Source: CAD feature listing. Evaluate the final solid. Frame: model axes, mm. A direction names the side the tool comes from. Give positions to 0.01 mm unless a question says otherwise; leave off trailing zeros. Loops run counter-clockwise (first coordinate to the right, second up) from the corner with the lowest first, then second, coordinate; pieces in that order, holes last. Notation, with made-up numbers: (15.25, 28.25) - (58.25, 28.25) arc R15 ccw to (58.25, 54.25) - close; hole circle Ø3 at (77.25, 88.25). An arc over 180 degrees is marked (long way). Put each result on its own line as item: value.
```python
from build123d import *

# Parameters (mm, degrees)
BOSS_EXTRUDE1_DEPTH = 5
SKETCH2_R           = 1.6
CUT_EXTRUDE1_DEPTH  = 3
BOSS_EXTRUDE2_DEPTH = 12
SKETCH8_R           = 1.5
CUT_EXTRUDE2_DEPTH  = 3
FILLET1_R           = 1
SKETCH9_W           = 6
SKETCH9_H           = 3
BOSS_EXTRUDE3_DEPTH = 5
SKETCH12_W          = 3
SKETCH12_H          = 5
CUT_EXTRUDE4_DEPTH  = 17
SKETCH14_W          = 4
SKETCH14_H          = 4
BOSS_EXTRUDE5_DEPTH = 6
FILLET3_R           = 4
FILLET4_R           = 4
BOSS_EXTRUDE6_DEPTH = 5


with BuildPart() as part:
    # Sketch1 → Boss-Extrude1 (new body)
    with BuildSketch(Plane(origin=(0, 0, 0), x_dir=(1, 0, 0), z_dir=(0, 1, 0))):
        Polygon((0, 0), (20, 0), (45, 12), (45, 22), (-25, 22), (-25, 12), align=None)
    extrude(amount=BOSS_EXTRUDE1_DEPTH)

    # Sketch2 → Cut-Extrude1 (cut)
    with BuildSketch(Plane(origin=(0, 5, 0), x_dir=(1, 0, 0), z_dir=(0, 1, 0))):
        with Locations(Location((4, 6, 0), (0, 0, 270))):
            Circle(SKETCH2_R)
        with Locations(Location((16, 6, 0), (0, 0, 90))):
            Circle(SKETCH2_R)
    extrude(amount=-CUT_EXTRUDE1_DEPTH, mode=Mode.SUBTRACT)

    # Sketch3 → Boss-Extrude2 (add)
    with BuildSketch(Plane(origin=(0, 5, 0), x_dir=(1, 0, 0), z_dir=(0, 1, 0))):
        with BuildLine():
            Line((-1.313075459, 8.787692444), (-14.45873126, 6.940191005))
            Line((-14.45873126, 6.940191005), (-25, 12))
            Line((-25, 12), (-25, 22))
            Line((-25, 22), (-22, 22))
            Line((-22, 22), (-22, 13.88770191))
            Line((-22, 13.88770191), (-13.978151779, 10.037214764))
            Line((-13.978151779, 10.037214764), (-3.068994172, 11.57039688))
            ThreePointArc((-3.068994172, 11.57039688), (0.071487045, 14.097332027), (4, 15))
            Line((4, 15), (16, 15))
            ThreePointArc((16, 15), (19.928512955, 14.097332027), (23.068994172, 11.57039688))
            Line((23.068994172, 11.57039688), (33.978151779, 10.037214764))
            Line((33.978151779, 10.037214764), (42, 13.88770191))
            Line((42, 13.88770191), (42, 22))
            Line((42, 22), (45, 22))
            Line((45, 22), (45, 12))
            Line((45, 12), (34.45873126, 6.940191005))
            Line((34.45873126, 6.940191005), (21.313075459, 8.787692444))
            ThreePointArc((21.313075459, 8.787692444), (19.104339329, 11.134498742), (16, 12))
            Line((16, 12), (4, 12))
            ThreePointArc((4, 12), (0.895660671, 11.134498742), (-1.313075459, 8.787692444))
        make_face()
    extrude(amount=BOSS_EXTRUDE2_DEPTH)

    # Sketch6 → Revolve1 (revolve)
    with BuildSketch(Plane.XY.offset(-6), mode=Mode.PRIVATE) as revolve1_sk:
        Polygon((2.4, 5), (2.4, 7), (1.4, 5), align=None)
    revolve(revolve1_sk.sketch.rotate(Axis((4, 5, -6), (0, 1, 0)), 270), axis=Axis((4, 5, -6), (0, 1, 0)))

    # Sketch7 → Revolve2 (revolve)
    with BuildSketch(Plane.XY.offset(-6), mode=Mode.PRIVATE) as revolve2_sk:
        Polygon((14.4, 5), (14.4, 7), (13.4, 5), align=None)
    revolve(revolve2_sk.sketch.rotate(Axis((16, 5, -6), (0, 1, 0)), 270), axis=Axis((16, 5, -6), (0, 1, 0)))

    # Sketch8 → Cut-Extrude2 (cut)
    with BuildSketch(Plane.XY.offset(-12)):
        with Locations((10, 11)):
            Circle(SKETCH8_R)
    extrude(amount=-CUT_EXTRUDE2_DEPTH, mode=Mode.SUBTRACT)

    # Fillet1
    fillet1_edges = [part.edges().sort_by_distance(p)[0] for p in [
        (8.5, 11, -15),
        (8.5, 11, -12),
    ]]
    fillet(fillet1_edges, radius=FILLET1_R)

    # Sketch9 → Boss-Extrude3 (add)
    with BuildSketch(Plane(origin=(0, 17, 0), x_dir=(1, 0, 0), z_dir=(0, 1, 0))):
        with Locations((10, 13.5)):
            Rectangle(SKETCH9_W, SKETCH9_H)
    extrude(amount=BOSS_EXTRUDE3_DEPTH)

    # Sketch12 → Cut-Extrude4 (cut)
    with BuildSketch(Plane(origin=(0, 17, 0), x_dir=(1, 0, 0), z_dir=(0, 1, 0))):
        with Locations((-23.5, 16.5)):
            Rectangle(SKETCH12_W, SKETCH12_H)
        with Locations((43.5, 16.5)):
            Rectangle(SKETCH12_W, SKETCH12_H)
    extrude(amount=-CUT_EXTRUDE4_DEPTH, mode=Mode.SUBTRACT)

    # Sketch14 → Boss-Extrude5 (add)
    with BuildSketch(Plane(origin=(0, 5, 0), x_dir=(1, 0, 0), z_dir=(0, 1, 0))):
        with Locations((34, 20)):
            Rectangle(SKETCH14_W, SKETCH14_H)
        with Locations((-14, 20)):
            Rectangle(SKETCH14_W, SKETCH14_H)
    extrude(amount=BOSS_EXTRUDE5_DEPTH)

    # Fillet3
    fillet3_edges = [part.edges().sort_by_distance(p)[0] for p in [
        (32, 8, -18),
    ]]
    fillet(fillet3_edges, radius=FILLET3_R - 0.0001)  # a hair under: the kernel refuses the full size

    # Fillet4
    fillet4_edges = [part.edges().sort_by_distance(p)[0] for p in [
        (-12, 8, -18),
    ]]
    fillet(fillet4_edges, radius=FILLET4_R - 0.0001)  # a hair under: the kernel refuses the full size

    # Sketch15 → Boss-Extrude6 (add)
    with BuildSketch(Plane(origin=(0, 5, 0), x_dir=(1, 0, 0), z_dir=(0, 1, 0))):
        Polygon((-16, 22), (-21, 29), (-1, 29), (-6, 22), align=None)
        Polygon((36, 22), (26, 22), (21, 29), (41, 29), align=None)
    extrude(amount=-BOSS_EXTRUDE6_DEPTH)


solid = part.part
```
1) Pin query (flat end, axial travel): P1, Ø3.5, axis at x = -24, z = -21, coming from the +Y side; P2, Ø1, axis at x = 20, y = 16.5, coming from the +Z side; P3, Ø3.5, axis at x = 20, z = -6.5, coming from the +Y side. Return the tip coordinate at first contact, or that it passes through.
Check result:
P1: y = 17
P2: z = -9.97
P3: y = 5.64
2) Section query C-C, the plane x = -18. Output: boundary loops of the cut face in (y, z), plus the area to 3 significant figures.
Check result:
outline: (0, -29) - (5, -29) - (5, -24.8) - (0, -24.8) - close; (0, -22) - (5, -22) - (5, -11.97) - (17, -11.97) - (17, -8.64) - (0, -8.64) - close
area: 128 mm²
3) Material intervals for line 1 along X through (y, z) = (5.4, -6); line 2 along Z through (x, y) = (4, 4.25); line 3 along X through (y, z) = (14.75, -13), sorted ascending. Write a range as [from, to].
Check result:
line 1: [1.6, 2.4], [5.6, 6.4], [13.6, 14.4], [17.6, 18.4]
line 2: [-22, -7.6], [-4.4, 0]
line 3: [-25, -20.15], [-1.66, 21.66], [40.15, 45]
4) Access query for faces 1 (the flat face through (37.933, 10.916, -11.936)), 2 (the flat face through (-24, 9, -19)), 3 (the flat face through (-14, 11, -20)), 4 (the flat face through (29, 17, -10)), 5 (the flat face through (31, 3, -29)). Directions: +Z, -Z, +X, -X, +Y, -Y. A direction counts if a zero-diameter tool reaches every point of the face in a straight line with its end or side. Return the directions, or none.
Check result:
face 1: +Y
face 2: -X, +Y, -Y
face 3: -Z, +Y
face 4: +Z, -Z, +X, +Y
face 5: -Z, +X, -X, +Y, -Y
5) Section query D-D, the plane z = -6. Output: boundary loops of the cut face in (x, y), plus the area to 3 significant figures.
Check result:
outline: (-12.5, 0) - (32.5, 0) - (32.5, 5) - (18.6, 5) - (17.6, 7) - (17.6, 2) - (14.4, 2) - (14.4, 7) - (13.4, 5) - (6.6, 5) - (5.6, 7) - (5.6, 2) - (2.4, 2) - (2.4, 7) - (1.4, 5) - (-12.5, 5) - close
area: 210 mm²
6) Section query B-B, the plane z = -23. Output: boundary loops of the cut face in (x, y).
Check result:
outline: (-16.71, 0) - (-5.29, 0) - (-5.29, 5) - (-16.71, 5) - close; (25.29, 0) - (36.71, 0) - (36.71, 5) - (25.29, 5) - close
7) Section query A-A, the plane y = 15.75. Output: boundary loops of the cut face in (x, z), plus the area to 3 significant figures.
Check result:
outline: (-25, -22) - (-22, -22) - (-22, -19) - (-25, -19) - close; (-25, -14) - (-22, -14) - (-22, -13.89) - (-13.98, -10.04) - (-3.07, -11.57) arc R9 ccw to (4, -15) - (16, -15) arc R9 ccw to (23.07, -11.57) - (33.98, -10.04) - (42, -13.89) - (42, -14) - (45, -14) - (45, -12) - (34.46, -6.94) - (21.31, -8.79) arc R6 cw to (16, -12) - (4, -12) arc R6 cw to (-1.31, -8.79) - (-14.46, -6.94) - (-25, -12) - close; (42, -22) - (45, -22) - (45, -19) - (42, -19) - close
area: 239 mm²
8) Mould query, pull axis Z, two halves, no side actions, for faces 6 (the flat face through (34, 8, -22)), 7 (the cylindrical face through (14.65, 4.54, -6.86)), 8 (the flat face through (-7.794, 10.916, -7.877)). Classes: pulls with the +Z half, pulls with the -Z half, needs draft (parallel to the pull), parting line crosses it, or undercut.
Check result:
face 6: pulls with the -Z half
face 7: undercut
face 8: pulls with the +Z half
